Geometry check sheet. Reference: the model listing, model coordinates, mm. A direction names the side the tool comes from. Round coordinates to 2 decimals unless told otherwise and drop trailing zeros. Order: outer loops, then holes, each group sorted by start corner. A loop starts at its lowest first (then second) coordinate and runs counter-clockwise, first axis right, second up. Notation, with made-up numbers: (-28.75, 55.25) -> (-5.75, 55.25) arc R9 cw to (-5.75, 69.25) -> close; hole circle Ø1 at (-28.5, 49). An arc over 180 degrees is marked (long way). Use a Markdown table: item, result. Add a question column.
Item 1: Sectioned sample at A-A, the plane z = 6.35. Record the cut outline in (x, y) (3 decimals).
Item 2: Gauge pin test, flat ends, axial feed: pin 1 Ø3 at (x, y) = (21, -2.5) entering from -Z; pin 2 Ø5 at (y, z) = (-6.5, 4) entering from +X (3 decimals); pin 3 Ø1 at (x, y) = (-2, 11.5) entering from +Z. Record the tip position at first contact, or that the pin passes through.
Item 3: Material ranges on probe 1 along Y at (x, z) = (14, 24) (3 decimals); probe 2 along Z at (x, y) = (20.5, -5.5) (3 decimals), recorded low to high. Write a range as [from, to].
Item 4: Set-up check for faces 5 (the flat face through (6, -15.875, 23)), 6 (the flat face through (15.875, 0, 5)), 7 (the flat face through (22, 0, 42.545)), 8 (the flat face through (22, 0, 44.45)), 9 (the flat face through (7, -13.97, 21)): record each of +Z, -Z, +X, -X, +Y, -Y from which the full face is reachable in a straight line by a thin tool's end or side.
Item 5: Sectioned sample at C-C, the plane x = 0. Record the cut outline in (y, z) (3 decimals), and give its area (3 significant figures).
Item 6: Sectioned sample at B-B, the plane y = 10.5. Record the cut outline in (x, z) (3 decimals).
Item 7: Sectioned sample at D-D, the plane z = 29.5. Record the cut outline in (x, y) (3 decimals).
Item 8: Mould release check, pull along X, two halves, no side actions. Record for faces 1 (the flat face through (-13.97, 0, 6)), 2 (the flat face through (22, 0, 14.605)), 3 (the cylindrical face through (16.599, 0.222, 11.936)), 4 (the flat face through (13.97, 0, 6)): pulls with the +X half, pulls with the -X half, needs draft (parallel to the pull), parting line crosses it, or undercut.
Autodesk Fusion 360 part; units mm, degrees
sketch "Sketch1" plane through (0, 0, 0) normal (0, 0, 1) x (1, 0, 0)
  line L0 (13.97, 13.97) -> (-13.97, 13.97)
  line L1 (-13.97, 13.97) -> (-13.97, -13.97)
  line L2 (-13.97, -13.97) -> (13.97, -13.97)
  line L3 (13.97, -13.97) -> (13.97, 13.97)
  line L4 (13.97, 13.97) -> (-13.97, -13.97) construction
  line L5 (-13.97, 13.97) -> (13.97, -13.97) construction
  line L6 (15.875, 15.875) -> (-15.875, 15.875)
  line L7 (-15.875, 15.875) -> (-15.875, -15.875)
  line L8 (-15.875, -15.875) -> (15.875, -15.875)
  line L9 (15.875, -15.875) -> (15.875, 15.875)
  line L10 (15.875, 15.875) -> (-15.875, -15.875) construction
  line L11 (-15.875, 15.875) -> (15.875, -15.875) construction
  dimension "d1" = 27.94
  dimension "d2" = 27.94
  dimension "d3" = 31.75
  dimension "d4" = 31.75
extrude "Extrude1" add sketch "Sketch1" along normal blind 12.7
revolve "Revolve1" add 1 faces at (-15.24, -4.6567, 12.7) angle 90 about axis through (15.875, -15.875, 12.7) along (0, 1, 0)
sketch "Sketch3" plane through (15.875, 0, 0) normal (1, 0, 0) x (0, 1, 0)
  line L0 (13.97, 14.605) -> (-13.97, 14.605)
  line L1 (-13.97, 14.605) -> (-13.97, 42.545)
  line L2 (-13.97, 42.545) -> (13.97, 42.545)
  line L3 (13.97, 42.545) -> (13.97, 14.605)
  line L4 (-15.875, 0) -> (15.875, 0)
  line L5 (15.875, 0) -> (15.875, 44.45)
  line L6 (15.875, 44.45) -> (-15.875, 44.45)
  line L7 (-15.875, 44.45) -> (-15.875, 0)
  line L8 (-13.97, 42.545) -> (13.97, 42.545)
  line L9 (13.97, 42.545) -> (13.97, 14.605)
  line L10 (13.97, 14.605) -> (-13.97, 14.605)
  line L11 (-13.97, 14.605) -> (-13.97, 42.545)
  line L12 (-15.875, 44.45) -> (14.2875, 44.45)
  line L13 (14.2875, 12.7) -> (-15.875, 12.7)
  line L14 (-15.875, 12.7) -> (-15.875, 44.45)
  line L15 (14.2875, 12.7) -> (15.875, 12.7)
  dimension "d10" = 31.75
extrude "Extrude2" add sketch "Sketch3" along normal blind 12.7 contours L5 L6 L7 L12 L13 L14 L15
fillet "Fillet1" radius 2.54 1 edges at (15.875, 0, 12.7)
sketch "Sketch5" plane through (0, 0, 12.7) normal (0, 0, -1) x (1, 0, 0)
  line L0 (18.415, 15.875) -> (18.415, -15.875)
  line L1 (18.415, -15.875) -> (28.575, -15.875)
  line L2 (28.575, -15.875) -> (28.575, 15.875)
  line L3 (28.575, 15.875) -> (18.415, 15.875)
sketch "Sketch6" plane through (0, -15.875, 0) normal (0, -1, 0) x (1, 0, 0)
  line L0 (-15.875, 0) -> (15.875, 0)
  line L1 (15.875, 0) -> (15.875, 10.16)
  arc A0 (18.415, 12.7) -> (15.875, 10.16) centre (18.415, 10.16) ccw
  line L2 (18.415, 12.7) -> (28.575, 12.7)
  line L3 (28.575, 12.7) -> (28.575, 44.45)
  line L4 (28.575, 44.45) -> (15.875, 44.45)
  arc A1 (15.875, 44.45) -> (-15.875, 12.7) centre (15.875, 12.7) ccw
  line L5 (-15.875, 12.7) -> (-15.875, 0)
  circle A2 centre (22.225, 28.575) radius 1.778
  line L6 (28.575, 12.7) -> (18.415, 12.7)
  dimension "d19" = 3.556
  dimension "d20" = 6.35
  dimension "d21" = 15.875
extrude "Extrude4" cut sketch "Sketch6" against normal blind 33.02 contours A2
sketch "Sketch7" plane through (0, -15.875, 0) normal (0, -1, 0) x (1, 0, 0)
  circle A0 centre (22.225, 28.575) radius 1.778
  line L0 (-15.875, 0) -> (15.875, 0)
  line L1 (15.875, 0) -> (15.875, 10.16)
  arc A1 (18.415, 12.7) -> (15.875, 10.16) centre (18.415, 10.16) ccw
  line L2 (18.415, 12.7) -> (28.575, 12.7)
  line L3 (28.575, 12.7) -> (28.575, 44.45)
  line L4 (28.575, 44.45) -> (15.875, 44.45)
  arc A2 (15.875, 44.45) -> (-15.875, 12.7) centre (15.875, 12.7) ccw
  line L5 (-15.875, 12.7) -> (-15.875, 0)
  circle A3 centre (0, 6.35) radius 1.778
  dimension "d24" = 3.556
  dimension "d25" = 6.35
  dimension "d26" = 15.875
extrude "Extrude5" cut sketch "Sketch7" against normal blind 35.56 contours A3
equation "d21 = ( 1.25 / 2 ) * 1 in"
Found:
| question | item | result |
|---|---|---|
| 1 | outline | (-15.875, -15.875) -> (-1.778, -15.875) -> (-1.778, -13.97) -> (-13.97, -13.97) -> (-13.97, 13.97) -> (-1.778, 13.97) -> (-1.778, 15.875) -> (-15.875, 15.875) -> close; (1.778, -15.875) -> (15.875, -15.875) -> (15.875, 15.875) -> (1.778, 15.875) -> (1.778, 13.97) -> (13.97, 13.97) -> (13.97, -13.97) -> (1.778, -13.97) -> close |
| 2 | pin 1 | stops at z = 12.7 |
| 2 | pin 2 | stops at x = 15.875 |
| 2 | pin 3 | stops at z = 39.27 |
| 3 | probe 1 | y = [-15.875, -13.97], [13.97, 15.875] |
| 3 | probe 2 | z = [12.7, 14.605], [42.545, 44.45] |
| 4 | face 5 | +Z, -Z, +X, -X, -Y |
| 4 | face 6 | -Z, +X, +Y, -Y |
| 4 | face 7 | +X |
| 4 | face 8 | +Z, +X, -X, +Y, -Y |
| 4 | face 9 | none |
| 5 | outline | (-15.875, 0) -> (-13.97, 0) -> (-13.97, 4.572) -> (-15.875, 4.572) -> close; (-15.875, 8.128) -> (-13.97, 8.128) -> (-13.97, 37.973) -> (13.97, 37.973) -> (13.97, 8.128) -> (15.875, 8.128) -> (15.875, 40.196) -> (-15.875, 40.196) -> close; (13.97, 0) -> (15.875, 0) -> (15.875, 4.572) -> (13.97, 4.572) -> close |
| 5 | area | 202 mm2 |
| 6 | outline | (-15.875, 0) -> (-13.97, 0) -> (-13.97, 12.7) arc R29.845 cw to (15.875, 42.545) -> (28.575, 42.545) -> (28.575, 44.45) -> (15.875, 44.45) arc R31.75 ccw to (-15.875, 12.7) -> close; (13.97, 0) -> (15.875, 0) -> (15.875, 10.16) arc R2.54 cw to (18.415, 12.7) -> (28.575, 12.7) -> (28.575, 14.605) -> (15.875, 14.605) arc R1.905 ccw to (13.97, 12.7) -> close |
| 7 | outline | (-11.066, -15.875) -> (20.707, -15.875) -> (20.707, -13.97) -> (-8.792, -13.97) -> (-8.792, 13.97) -> (20.707, 13.97) -> (20.707, 15.875) -> (-11.066, 15.875) -> close; (23.743, -15.875) -> (28.575, -15.875) -> (28.575, -13.97) -> (23.743, -13.97) -> close; (23.743, 13.97) -> (28.575, 13.97) -> (28.575, 15.875) -> (23.743, 15.875) -> close |
| 8 | face 1 | undercut |
| 8 | face 2 | needs draft |
| 8 | face 3 | pulls with the +X half |
| 8 | face 4 | undercut |
